from build123d import *

# Parameters (mm, degrees)
BOSS_EXTRUDE1_DEPTH   = 3.175
M4X0_7_TAPPED_HOLE1_D = 3.3
M4_CLEARANCE_HOLE1_D  = 4.5


with BuildPart() as part:
    # Sketch1 → Boss-Extrude1 (new body, symmetric)
    with BuildSketch(Plane(origin=(0, 0, 0), x_dir=(1, 0, 0), z_dir=(0, 1, 0))):
        Polygon((0, 0), (0, 20), (4, 26.363068172), (19, 26.363068172), (19, 16.363068172), (7.5, 0), align=None)
    extrude(amount=BOSS_EXTRUDE1_DEPTH, both=True)

    # M4x0.7 Tapped Hole1 (through all)
    with Locations(Plane(origin=(0, 3.175, 0), x_dir=(1, 0, 0), z_dir=(0, 1, 0))):
        with Locations((4.499999553, 15), (4.499999553, 5)):
            Hole(M4X0_7_TAPPED_HOLE1_D / 2)

    # M4 Clearance Hole1 (through all)
    with Locations(Plane(origin=(0, 3.175, 0), x_dir=(1, 0, 0), z_dir=(0, 1, 0))):
        with Locations((11.5, 21.364471274)):
            Hole(M4_CLEARANCE_HOLE1_D / 2)


solid = part.part
Geometry check sheet. Reference: the model listing, model coordinates, mm. Coordinates: 2 decimals unless noted, no trailing zeros. Order: outer loops, then holes, each group sorted by start corner. A loop starts at its lowest first (then second) coordinate and runs counter-clockwise, first axis right, second up. Notation, with made-up numbers: (13, 74.25) - (25, 74.25) arc R31 cw to (25, 109.25) - close; hole circle Ø7 at (66, 83). An arc over 180 degrees is marked (long way). Answer in a Markdown table with one row per item. Add a question column.
1) Cross-section at A-A, the plane x = 4.5. Record the cut outline in (y, z) (3 decimals).
2) Release check for a two-part mould opening along Z. For faces 1 (the flat face through (10, -3.175, -16)), 2 (the cylindrical face through (11.793, -0.044, -23.595)), 3 (the flat face through (1.972, 0.044, -23.137)) record: +Z half, -Z half, draft (parallel to the pull), parting line (faces both ways), or undercut.
3) Material ranges on line 1 along Z through (x, y) = (4.5, 1); line 2 along X through (y, z) = (0.5, -21.5); line 3 along X through (y, z) = (-1, -15), recorded low to high. Write a range as [from, to].
4) Cross-section at D-D, the plane x = 12.25. Record the cut outline in (y, z) (3 decimals).
5) Gauge pin test, flat ends, axial feed: P1, Ø3, axis at x = 14, z = -6.5, coming from the -Y side; P2, Ø2, axis at y = -2.5, z = -20.5, coming from the -X side. Record the tip position at first contact, or that the pin passes through.
6) Cross-section at B-B, the plane z = -6. Record the cut outline in (x, y) (3 decimals), then the cut area to 3 significant figures.
7) Cross-section at C-C, the plane y = -0.75. Record the cut outline in (x, z), then the cut area to 3 significant figures.
Check result:
| question | item | result |
|---|---|---|
| 1 | outline | (-3.175, -26.363) - (3.175, -26.363) - (3.175, -16.65) - (-3.175, -16.65) - close; (-3.175, -13.35) - (3.175, -13.35) - (3.175, -6.65) - (-3.175, -6.65) - close; (-3.175, -3.35) - (3.175, -3.35) - (3.175, 0) - (-3.175, 0) - close |
| 2 | face 1 | draft |
| 2 | face 2 | undercut |
| 2 | face 3 | -Z half |
| 3 | line 1 | z = [-26.36, -16.65], [-13.35, -6.65], [-3.35, 0] |
| 3 | line 2 | x = [0.94, 9.25], [13.75, 19] |
| 3 | line 3 | x = [0, 2.85], [6.15, 18.04] |
| 4 | outline | (-3.175, -26.363) - (3.175, -26.363) - (3.175, -23.486) - (-3.175, -23.486) - close; (-3.175, -19.243) - (3.175, -19.243) - (3.175, -6.759) - (-3.175, -6.759) - close |
| 5 | P1 | passes through |
| 5 | P2 | stops at x = 0 |
| 6 | outline | (0, -3.175) - (3.188, -3.175) - (3.188, 3.175) - (0, 3.175) - close; (5.812, -3.175) - (11.717, -3.175) - (11.717, 3.175) - (5.812, 3.175) - close |
| 6 | area | 57.7 mm² |
| 7 | outline | (0, -20) - (4, -26.36) - (19, -26.36) - (19, -16.36) - (7.5, 0) - (0, 0) - close; hole circle Ø3.3 at (4.5, -15); hole circle Ø3.3 at (4.5, -5); hole circle Ø4.5 at (11.5, -21.36) |
| 7 | area | 361 mm² |
